Here's how the part is built. I have some questions about the finished solid (model axes, mm). A direction names the side the tool comes from. Round coordinates to 2 decimals unless told otherwise and drop trailing zeros. Write each loop counter-clockwise with the first axis right and the second up, starting at its lowest first coordinate (ties: lowest second). Pieces come first, ordered by that corner, then holes. Notation, with made-up numbers: M 86.25,63 L 102.25,63 A8 cw 102.25,72 Z; hole C -26,-18 d9. An arc over 180 degrees is marked long. Use one line per item in the form item = value. Start each with the question number.
Q1. I want a section at B-B on x = 20. List the corners of the cut face in (y, z) for me (3 decimals).
Q2. I'm going to push flat-ended pins straight in: pin 1 Ø15.5 at (x, y) = (0, 17.399) entering from -Z; pin 2 Ø9 at (x, y) = (0, 17.399) entering from -Z; pin 3 Ø6 at (x, y) = (23.876, -30.226) entering from -Z. Where does each tip first touch, or does it pass through?
Q3. I want a section at A-A on y = 28. State how many separate pieces and enclosed holes the cut face has, and give its area (3 significant figures).
Q4. We'd pull the mould along Y, two halves only. Please class faces 3 (the face through (-2.759, 4.976, -17.66)), 4 (the face through (0, 41.275, 0)), 5 (the face through (0, -1, 19.05)): +Y half, -Y half, draft (parallel to the pull), parting line (faces both ways), or undercut.
Q5. I want a section at D-D on x = 0. List the corners of the cut face in (y, z) for me (3 decimals), and give its area (3 significant figures).
Q6. For faces 1 (the face through (0, -18, 9.398)), 2 (the face through (0, -1, -19.05)), which set-ups out of +Z, -Z, +X, -X, +Y, -Y let a thin tool reach every point of the face, with its end or its side?
Q7. I want a section at C-C on z = 4.5. List the corners of the cut face in (x, y) for me (3 decimals), and give its area (3 significant figures).
Q8. I need wall thicknesses on line 1 along Y through (x, z) = (0, -17.7) (3 decimals); line 2 along X through (y, z) = (17.5, -16) (1 decimal); line 3 along X through (y, z) = (33, 4.5) (3 decimals). Which ranges of each line are inside material? Lowest first, please. Write a range as from..to.
```python
from build123d import *

# Parameters (mm, degrees)
SKETCH1_W           = 82.55
SKETCH1_H           = 69.85
BOSS_EXTRUDE1_DEPTH = 19.05
CUT_EXTRUDE2_START  = -19.05
SKETCH2_R           = 5.159375
CUT_EXTRUDE2_DEPTH  = 38.1
CUT_EXTRUDE4_START  = -19.05
SKETCH3_R           = 5.159375
CUT_EXTRUDE4_DEPTH  = 38.1
CUT_EXTRUDE6_START  = -19.05
SKETCH4_R           = 7.3421875
CUT_EXTRUDE6_DEPTH  = 28.448
CUT_EXTRUDE8_START  = -19.05
SKETCH5_R           = 12.7254
CUT_EXTRUDE8_DEPTH  = 2.8194
CUT_EXTRUDE10_START = -19.05
SKETCH6_R           = 7.3421875
CUT_EXTRUDE10_DEPTH = 28.448
CUT_EXTRUDE12_START = -19.05
SKETCH7_R           = 12.7254
CUT_EXTRUDE12_DEPTH = 2.8194


with BuildPart() as part:
    # Sketch1 → Boss-Extrude1 (new, symmetric)
    with BuildSketch(Plane(origin=(0, 0, 0), x_dir=(0, 1, 0), z_dir=(0, 0, 1))):
        Rectangle(SKETCH1_W, SKETCH1_H)
    extrude(amount=BOSS_EXTRUDE1_DEPTH, both=True)

    # Sketch2 → Cut-Extrude2 (cut)
    with BuildSketch(Plane(origin=(0, 0, 0), x_dir=(0, 1, 0), z_dir=(0, 0, 1)).offset(CUT_EXTRUDE2_START)):
        with Locations(Location((-30.226, -23.876, 0), (0, 0, 90))):
            Circle(SKETCH2_R)
    extrude(amount=CUT_EXTRUDE2_DEPTH, mode=Mode.SUBTRACT)

    # Sketch3 → Cut-Extrude4 (cut)
    with BuildSketch(Plane(origin=(0, 0, 0), x_dir=(0, 1, 0), z_dir=(0, 0, 1)).offset(CUT_EXTRUDE4_START)):
        with Locations(Location((30.099, -23.876, 0), (0, 0, 90))):
            Circle(SKETCH3_R)
        with Locations(Location((-30.226, 23.749, 0), (0, 0, 90))):
            Circle(SKETCH3_R)
        with Locations(Location((30.099, 23.749, 0), (0, 0, 90))):
            Circle(SKETCH3_R)
    extrude(amount=CUT_EXTRUDE4_DEPTH, mode=Mode.SUBTRACT)

    # Sketch4 → Cut-Extrude6 (cut)
    with BuildSketch(Plane(origin=(0, 0, 0), x_dir=(0, 1, 0), z_dir=(0, 0, 1)).offset(CUT_EXTRUDE6_START)):
        with Locations(Location((-17.653, 0, 0), (0, 0, 270))):
            Circle(SKETCH4_R)
    extrude(amount=CUT_EXTRUDE6_DEPTH, mode=Mode.SUBTRACT)

    # Sketch5 → Cut-Extrude8 (cut)
    with BuildSketch(Plane(origin=(0, 0, 0), x_dir=(0, 1, 0), z_dir=(0, 0, 1)).offset(CUT_EXTRUDE8_START)):
        with Locations(Location((-17.653, 0, 0), (0, 0, 270))):
            Circle(SKETCH5_R)
    extrude(amount=CUT_EXTRUDE8_DEPTH, mode=Mode.SUBTRACT)

    # Sketch6 → Cut-Extrude10 (cut)
    with BuildSketch(Plane(origin=(0, 0, 0), x_dir=(0, 1, 0), z_dir=(0, 0, 1)).offset(CUT_EXTRUDE10_START)):
        with Locations(Location((17.399, 0, 0), (0, 0, 270))):
            Circle(SKETCH6_R)
    extrude(amount=CUT_EXTRUDE10_DEPTH, mode=Mode.SUBTRACT)

    # Sketch7 → Cut-Extrude12 (cut)
    with BuildSketch(Plane(origin=(0, 0, 0), x_dir=(0, 1, 0), z_dir=(0, 0, 1)).offset(CUT_EXTRUDE12_START)):
        with Locations(Location((17.399, 0, 0), (0, 0, 270))):
            Circle(SKETCH7_R)
    extrude(amount=CUT_EXTRUDE12_DEPTH, mode=Mode.SUBTRACT)


solid = part.part
```
Reported:
q1.outline = M -41.275,-19.05 L -33.631,-19.05 L -33.631,19.05 L -41.275,19.05 Z; M -26.821,-19.05 L 26.694,-19.05 L 26.694,19.05 L -26.821,19.05 Z; M 33.504,-19.05 L 41.275,-19.05 L 41.275,19.05 L 33.504,19.05 Z
q2.pin_1 = -16.23
q2.pin_2 = 9.4
q2.pin_3 = through
q3.separate_pieces = 3
q3.enclosed_holes = 0
q3.area = 1,900 mm^2
q4.face_3 = undercut
q4.face_4 = +Y half
q4.face_5 = draft
q5.outline = M -41.275,-19.05 L -30.378,-19.05 L -30.378,-16.231 L -24.995,-16.231 L -24.995,9.398 L -10.311,9.398 L -10.311,-16.231 L -4.928,-16.231 L -4.928,-19.05 L 4.674,-19.05 L 4.674,-16.231 L 10.057,-16.231 L 10.057,9.398 L 24.741,9.398 L 24.741,-16.231 L 30.124,-16.231 L 30.124,-19.05 L 41.275,-19.05 L 41.275,19.05 L -41.275,19.05 Z
q5.area = 2,250 mm^2
q6.face_1 = -Z
q6.face_2 = -Z, +X, -X, +Y, -Y
q7.outline = M -34.925,-41.275 L 34.925,-41.275 L 34.925,41.275 L -34.925,41.275 Z; hole C -23.749,-30.226 d10.319; hole C -23.749,30.099 d10.319; hole C 0,-17.653 d14.684; hole C 0,17.399 d14.684; hole C 23.876,-30.226 d10.319; hole C 23.876,30.099 d10.319
q7.area = 5,090 mm^2
q8.line_1 = -41.275..-30.378, -4.928..4.674, 30.124..41.275
q8.line_2 = -34.9..-7.3, 7.3..34.9
q8.line_3 = -34.925..-28.016, -19.482..19.609, 28.143..34.925
